Autodesk Inventor part; units mm, degrees
ref_plane "YZ Plane" through (0, 0, 0) normal (1, 0, 0) x (0, 1, 0)
ref_plane "XZ Plane" through (0, 0, 0) normal (0, 1, 0) x (-1, 0, 0)
ref_plane "XY Plane" through (0, 0, 0) normal (0, 0, 1) x (1, 0, 0)
sketch "Sketch1" plane through (0, 0, 0) normal (0, 0, 1) x (1, 0, 0)
  circle A0 centre (0, 0) radius 11.11
  arc A1 (-31.75, 0) -> (31.75, 0) centre (0, 0) ccw
  line L0 (31.75, 0) -> (31.75, 52.4)
  line L1 (-31.75, 0) -> (-31.75, 52.4)
  line L2 (-31.75, 74.62) -> (31.75, 74.62) construction
  line L3 (-31.75, 112.4) -> (31.75, 112.4)
  line L4 (31.75, 52.4) -> (31.75, 112.4)
  line L5 (-31.75, 112.4) -> (-31.75, 52.4)
  point P0 (0, 74.62)
  dimension "d0" = 22.22
  dimension "d3" = 31.75
  dimension "d4" = 52.4
  dimension "d7" = 74.62
  dimension "d17" = 60
extrude "Extrusion1" add sketch "Sketch1" along normal mid plane 70
sketch "Sketch2" plane through (0, 0, 0) normal (1, 0, 0) x (0, 1, 0)
  line L0 (52.4, 14.3) -> (-52.4, 14.3)
  line L1 (-52.4, 14.3) -> (-52.4, -14.3)
  line L2 (-52.4, -14.3) -> (52.4, -14.3)
  line L3 (52.4, -14.3) -> (52.4, 14.3)
  line L4 (52.4, 14.3) -> (-52.4, -14.3) construction
  line L5 (-52.4, 14.3) -> (52.4, -14.3) construction
  point P0 (0, 0)
  dimension "d13" = 28.6
  dimension "d14" = 52.4
extrude "Extrusion2" cut sketch "Sketch2" along normal through all both and the other way through all
sketch "Sketch3" plane through (0, 0, 0) normal (1, 0, 0) x (0, 1, 0)
  line L0 (52.4, 14.3) -> (52.4, -14.3)
  line L1 (112.4, -35) -> (112.4, 35)
  line L2 (52.4, 14.3) -> (52.4, 35)
  line L3 (52.4, -14.3) -> (52.4, -35)
  line L4 (52.4, 0) -> (112.4, 0)
  line L5 (112.4, -35) -> (112.4, -45)
  line L6 (52.4, -35) -> (52.4, -45)
  line L7 (52.4, 35) -> (52.4, 45)
  line L8 (112.4, 35) -> (112.4, 45)
  arc A0 (52.4, -45) -> (112.4, -45) centre (82.4, -35) ccw
  line L9 (112.4, -35) -> (0, -35)
  arc A1 (112.4, 45) -> (52.4, 45) centre (82.4, 35) ccw
  point P0 (0, 0)
  dimension "d22" = 10
sketch "Sketch4" plane through (-31.75, 112.4, 35) normal (0, 1, 0) x (1, 0, 0)
  line L0 (0, 70) -> (0, 0)
  line L1 (63.5, 0) -> (0, 0)
  line L2 (63.5, 70) -> (63.5, 0)
  line L3 (0, 70) -> (63.5, 70)
  line L4 (15, 15) -> (15, 55)
  line L5 (15, 55) -> (48.5, 55)
  line L6 (48.5, 55) -> (48.5, 15)
  line L7 (48.5, 15) -> (15, 15)
  point P0 (31.75, 35)
  dimension "d19" = 15
extrude "Extrusion3" cut sketch "Sketch4" against normal up to surface (60 mm away)
revolve "Revolution1" add sketch "Sketch3" angle 360 about axis through (0, 52.4, 0) along (0, 1, 0) contours L2 L7 A1 L8 L1 L4 L0
chamfer "Chamfer1" distance 5 angle 45 6 edges at (31.75, 26.2, 35) (0, -31.75, 35) (-31.75, 26.2, 35) (31.75, 26.2, -35) (0, -31.75, -35) (-31.75, 26.2, -35)
sketch "Sketch5" plane through (0, 0, 0) normal (0, 0, 1) x (1, 0, 0)
  line L0 (31.75, 52.4) -> (31.75, 0)
  line L1 (31.75, 52.4) -> (91.75, 52.4)
  line L2 (91.75, 52.4) -> (91.75, 112.4)
  line L3 (91.75, 112.4) -> (31.75, 112.4)
  line L4 (31.75, 112.4) -> (31.75, 52.4)
  line L5 (45, 112.4) -> (-45, 112.4) construction
  line L6 (0, 52.4) -> (0, 112.4)
  line L7 (-31.75, 52.4) -> (-31.75, 0)
  line L8 (-31.75, 52.4) -> (-91.75, 52.4)
  line L9 (-91.75, 52.4) -> (-91.75, 112.4)
  line L10 (-91.75, 112.4) -> (-31.75, 112.4)
  line L11 (-31.75, 112.4) -> (-31.75, 52.4)
  line L12 (-45, 112.4) -> (45, 112.4) construction
  point P0 (0, 0)
  dimension "d28" = 60
extrude "Extrusion4" cut sketch "Sketch5" along normal through all both and the other way through all
sketch "Sketch6" plane through (0, 0, 0) normal (1, 0, 0) x (0, 1, 0)
  line L0 (112.4, 31.8895) -> (112.4, -31.8895)
  line L1 (112.4, 0) -> (112.4, 15)
  line L2 (112.4, 15) -> (97.4, 15)
  arc A0 (97.4, 15) -> (67.4, 15) centre (82.4, 15) ccw
  line L3 (112.4, 0) -> (67.4, 0)
  line L4 (67.4, 0) -> (67.4, 15)
  point P0 (0, 0)
  dimension "d31" = 15
  dimension "d32" = 15
  dimension "d34" = 15
revolve "Revolution2" cut sketch "Sketch6" angle 360 about axis through (0, 112.4, 0) along (0, -1, 0)
sketch "Sketch7" plane through (31.75, 0, 14.3) normal (1, 0, 0) x (0, 0, -1)
  line L0 (29.3, 67.4) -> (-0.7, 67.4)
  line L1 (29.3, 97.4) -> (-0.7, 97.4) construction
  arc A0 (-0.7, 97.4) -> (-0.7, 67.4) centre (-0.7, 82.4) ccw
  arc A1 (29.3, 67.4) -> (29.3, 97.4) centre (29.3, 82.4) ccw
  line L2 (46.1895, 112.4) -> (-17.5895, 112.4) construction
  line L3 (29.3, 112.4) -> (29.3, 97.4)
  line L4 (29.3, 112.4) -> (-0.7, 112.4)
  line L5 (-0.7, 97.4) -> (-0.7, 112.4)
  point P0 (14.3, 0)
extrude "Extrusion5" cut sketch "Sketch7" against normal up to surface (31.75 mm away)
properties part number "Clevis-Socket"
Check sheet for the modelled part. Datum: model origin and axes. Units: mm. A direction names the side the tool comes from. Give positions to 0.01 mm unless a question says otherwise; leave off trailing zeros. Order: outer loops, then holes, each group sorted by start corner. A loop starts at its lowest first (then second) coordinate and runs counter-clockwise, first axis right, second up. Notation, with made-up numbers: M 63.5,8.25 L 85.5,8.25 A18 ccw 85.5,39.25 Z; hole C 44.5,22 d8. An arc over 180 degrees is marked long. Answer as CSV lines item,"result". Start each with the question number.
Item 1: Cross-section at B-B on x = -6. State how many separate pieces and enclosed holes the cut face has, plus the area to 3 significant figures.
Item 2: Cross-section at A-A on y = 27. Enter the section's corners in (x, z).
Item 3: Gauge pin test, flat ends, axial feed: P1, Ø8, axis at x = -12, y = 85.5, coming from the +Z side; P2, Ø6, axis at x = -5, y = 38, coming from the +Z side; P3, Ø12, axis at x = 14, y = 73.5, coming from the +Z side. Record the tip position at first contact, or that the pin passes through.
Item 4: Tool access check on faces 4 (the face through (29.28, 25.83, 32.47)), 5 (the face through (-29.28, 25.83, 32.47)), 6 (the face through (29.28, 25.83, -32.47)), 7 (the face through (0, 52.4, 0)), 8 (the face through (-15, 105, 0)). Record the directions out of +Z, -Z, +X, -X, +Y, -Y that give a thin tool (end or side, any length) a straight path to the whole face; none if there is none.
Item 5: Thickness scan on line 1 (Z direction, x = 10.5, y = 19.5); line 2 (Y direction, x = 1, z = -26.5); line 3 (X direction, y = 0, z = 28). Record the ranges inside material, lowest first. Write a range as [from, to].
Item 6: Mould release check, pull along Y, two halves, no side actions. Record for faces 1 (the face through (0, 13, 35)), 2 (the face through (-8.817, 6.76, -24.795)), 3 (the face through (0, 52.4, -39)): +Y half, -Y half, draft (parallel to the pull), parting line (faces both ways), or undercut.
Established:
1,separate pieces,"3"
1,enclosed holes,"0"
1,area,"7,940 mm^2"
2,outline,"M -31.75,-30 L -26.75,-35 L 26.75,-35 L 31.75,-30 L 31.75,-14.3 L -31.75,-14.3 Z; M -31.75,14.3 L 31.75,14.3 L 31.75,30 L 26.75,35 L -26.75,35 L -31.75,30 Z"
3,P1,"stops at z = 66.06"
3,P2,"stops at z = 35"
3,P3,"stops at z = 65.56"
4,face 4,"+Z, +X, -Y"
4,face 5,"+Z, -X, -Y"
4,face 6,"-Z, +X, -Y"
4,face 7,"+X, -X, -Y"
4,face 8,"+X, +Y"
5,line 1,"z = [-35, -14.3], [14.3, 35]"
5,line 2,"y = [-31.73, -11.06], [11.06, 72.77], [92.03, 112.4]"
5,line 3,"x = [-31.75, -11.11], [11.11, 31.75]"
6,face 1,"draft"
6,face 2,"undercut"
6,face 3,"-Y half"
